For this review, take the finished solid that the model builds, in its own axes (mm). Give positions to 0.01 mm unless a question says otherwise; leave off trailing zeros. Write each loop counter-clockwise with the first axis right and the second up, starting at its lowest first coordinate (ties: lowest second). Pieces come first, ordered by that corner, then holes. Notation, with made-up numbers: (63.5, -23) -> (103.5, -23) arc R18 ccw to (103.5, 11) -> close; hole circle Ø4 at (63.5, 15). An arc over 180 degrees is marked (long way). Return JSON: item names as keys, results as strings.
Autodesk Fusion 360 part; units mm, degrees
sketch "Sketch tranche" plane through (0, 0, 0) normal (0, 0, 1) x (1, 0, 0)
  line L0 (0, 0) -> (1.5, 0)
  line L1 (1.5, 0) -> (1.5, 17)
  line L2 (1.5, 17) -> (0, 17)
  line L3 (0, 17) -> (0, 0)
  line L4 (7.75, 0) -> (7.75, 16)
  line L5 (1.5, 17) -> (-3, 17)
  line L6 (-3, 17) -> (-3, 19)
  line L7 (-3, 19) -> (1.5, 19)
  line L8 (1.5, 19) -> (1.5, 17)
  dimension "d1" = 1.5
  dimension "d2" = 17
  dimension "d3" = 7.75
  dimension "d4" = 3
  dimension "d5" = 2
revolve "Revolve1" add sketch "Sketch tranche" angle 360 about axis through (7.75, 0, 0) along (0, 1, 0)
1. Add section C-C, the plane y = 2.5. State the section outline as (x, z) points, plus the area to 3 significant figures.
Results found:
{"outline": "circle Ø15.5 at (7.75, 0); hole circle Ø12.5 at (7.75, 0)", "area": "66.0 mm²"}
2. Add section A-A, the plane z = 0. State the section outline as (x, y) points, plus the area to 3 significant figures.
Results found:
{"outline": "(-3, 17) -> (0, 17) -> (0, 0) -> (1.5, 0) -> (1.5, 19) -> (-3, 19) -> close; (14, 0) -> (15.5, 0) -> (15.5, 17) -> (18.5, 17) -> (18.5, 19) -> (14, 19) -> close", "area": "69.0 mm²"}
3. The part is to be moulded in two halves that separate along X. For faces 1 (the cylindrical face through (12.71, 9.37, 3.8)), 2 (the flat face through (2, 17, 6)), 3 (the cylindrical face through (15.493, 8.381, -0.341)), say which applies: +X half, -X half, draft (parallel to the pull), parting line (faces both ways), or undercut.
Results found:
{"face 1": "undercut", "face 2": "draft", "face 3": "parting line"}
4. Add section D-D, the plane x = -1.5. State the section outline as (y, z) points.
Results found:
{"outline": "(17, -5.48) -> (19, -5.48) -> (19, 5.48) -> (17, 5.48) -> close"}
5. Add section B-B, the plane x = 7.75. State the section outline as (y, z) points, plus the area to 3 significant figures.
Results found:
{"outline": "(0, -7.75) -> (17, -7.75) -> (17, -10.75) -> (19, -10.75) -> (19, -6.25) -> (0, -6.25) -> close; (0, 6.25) -> (19, 6.25) -> (19, 10.75) -> (17, 10.75) -> (17, 7.75) -> (0, 7.75) -> close", "area": "69.0 mm²"}
6. To check wall thickness, follow probe 1 along X at (y, z) = (8.5, -0.25) (3 decimals); probe 2 along Z at (x, y) = (7.75, 10.5); probe 3 along Y at (x, z) = (14, 5.75). State the ranges of each line that lie inside material, in increasing order.
Results found:
{"probe 1": "x = 0.004 to 1.505, 13.995 to 15.496", "probe 2": "z = -7.75 to -6.25, 6.25 to 7.75", "probe 3": "y = 17 to 19"}
7. For pin 1 (6 mm diameter, centred on y = 9, z = -7.5, fed in from +X); pin 2 (5 mm diameter, centred on x = 4.5, y = 10, fed in from +Z); pin 3 (6 mm diameter, centred on y = 6.5, z = 8, fed in from +X), all flat-tipped, find the tip position at first contact; note any pin that passes through.
Results found:
{"pin 1": "stops at x = 14.06", "pin 2": "stops at z = 7.71", "pin 3": "stops at x = 13.67"}
